Print and shaded views of the part. All mm, measured from the part's lowest x, y and z. A direction names the side the tool comes from. Round coordinates to 2 decimals unless told otherwise and drop trailing zeros. Order: outer loops, then holes, each group sorted by start corner. A loop starts at its lowest first (then second) coordinate and runs counter-clockwise, first axis right, second up. Notation, with made-up numbers: (23.25, -15.75) - (68.25, -15.75) arc R24 ccw to (68.25, 21.25) - close; hole circle Ø2 at (81, 31.5). An arc over 180 degrees is marked (long way). Write item = value, one per line. Start each with the question number.
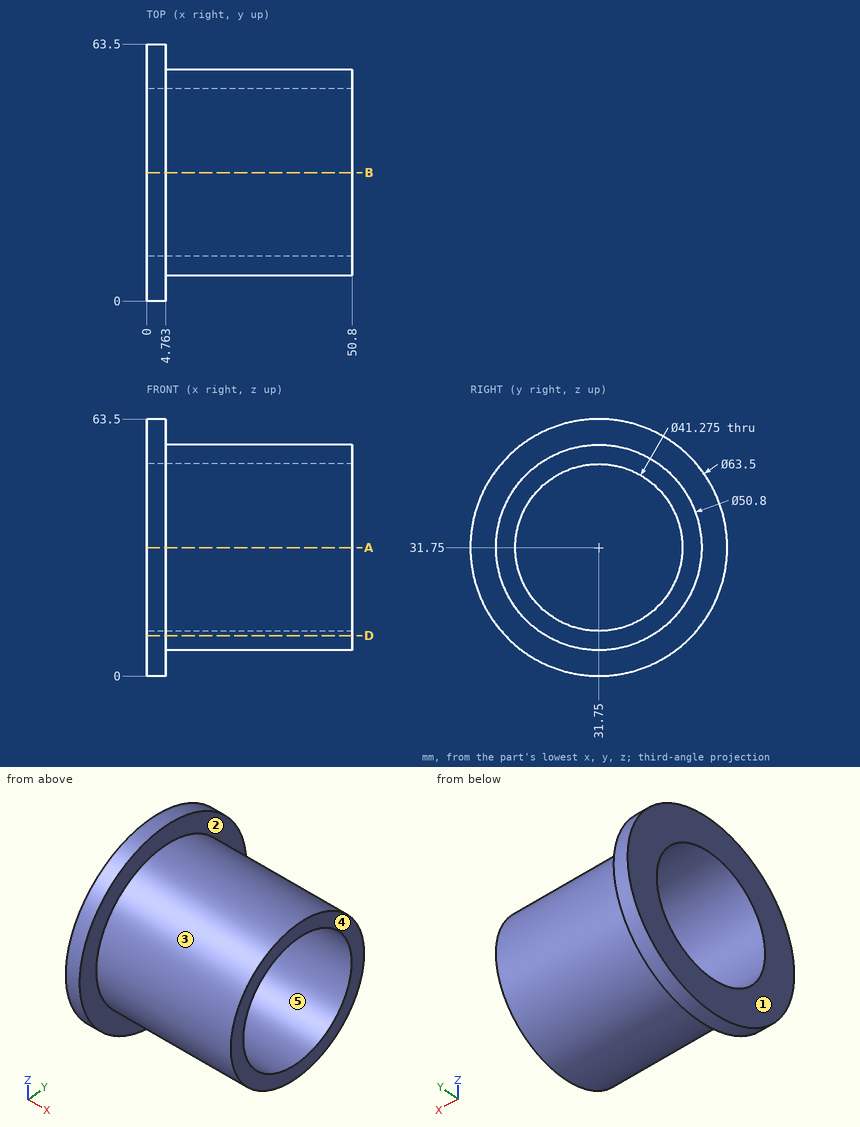
Item 1: Saw through at D-D, the plane z = 10. Give the cut face in (x, y), then the cut area to 3 significant figures.
Item 2: Drop flat-ended pins along their axis: pin 1 (4 mm diameter, centred on x = 30.5, y = 38.5, fed in from +Z); pin 2 (1 mm diameter, centred on y = 50.5, z = 9.5, fed in from +X); pin 3 (10 mm diameter, centred on x = 28.5, z = 14, fed in from +Y). Give the stop position or say it passes through.
Item 3: Probe L1, parallel to Z at x = 23, y = 31; L2, parallel to X at y = 11.5, z = 8.5. List the from-to ranges inside material, lowest first.
Item 4: Which spindle directions (+Z, -Z, +X, -X, +Y, -Y) get a long thin tool onto all of the face, cutting with end or side? Do the marked faces 1 and 2. Say none if no direction does.
Item 5: Mould opens along Y. For the marked faces 3, 4 and 5 say: +Y half, -Y half, draft (parallel to the pull), parting line (faces both ways), or undercut.
Item 6: Saw through at A-A, the plane z = 31.75. Give the cut face in (x, y).
Check sheet entries:
q1.outline = (0, 8.62) - (4.76, 8.62) - (4.76, 18.63) - (50.8, 18.63) - (50.8, 44.87) - (4.76, 44.87) - (4.76, 54.88) - (0, 54.88) - close
q1.area = 1,430 mm2
q2.pin_1 = 56.7
q2.pin_2 = 4.76
q2.pin_3 = 53.72
q3.L1 = 6.36 to 11.13, 52.37 to 57.14
q3.L2 = 0 to 4.76
q4.face_1 = +Z, -Z, -X, +Y, -Y
q4.face_2 = +X
q5.face_3 = parting line
q5.face_4 = draft
q5.face_5 = undercut
q6.outline = (0, 0) - (4.76, 0) - (4.76, 6.35) - (50.8, 6.35) - (50.8, 11.11) - (0, 11.11) - close; (0, 52.39) - (50.8, 52.39) - (50.8, 57.15) - (4.76, 57.15) - (4.76, 63.5) - (0, 63.5) - close
